For this review, take the finished solid that the model builds, in its own axes (mm). A direction names the side the tool comes from. Coordinates: 2 decimals unless noted, no trailing zeros. Loops run counter-clockwise (first coordinate to the right, second up) from the corner with the lowest first, then second, coordinate; pieces in that order, holes last. Notation, with made-up numbers: (48, -12.75) - (95, -12.75) arc R31 cw to (95, 26.25) - close; hole circle Ø11 at (9, 85). An arc over 180 degrees is marked (long way). One line per item, written item: value. Start each with the question number.
1. For faces 5 (the face through (37, 0, -5)), 6 (the face through (41, 0, -7.5)), 7 (the face through (37, 5, 0)), 8 (the face through (2.8, -8, 0)), 9 (the face through (7, 7, 2.5)), list the 3-axis set-ups (+Z, -Z, +X, -X, +Y, -Y) from which the entire face can be reached by the end or side of a thin tool; tool diameter is ignored.
2. Insertion check: pin 1 (2.5 mm diameter, centred on y = -8, z = 0.5, fed in from +X); pin 2 (4 mm diameter, centred on x = 17, y = 8.5, fed in from -Z); pin 3 (2.5 mm diameter, centred on x = 37.5, z = -0.5, fed in from -Y). Each pin has a flat end and moves straight along its axis. Give the tip position at first contact, or say it passes through.
3. Take a section at D-D, the plane x = 31.5. State the section outline as (y, z) points.
4. Take a section at A-A, the plane x = 0. State the section outline as (y, z) points.
5. Take a section at C-C, the plane y = 2. State the section outline as (x, z) points, and give its area (3 significant figures).
6. Take a section at B-B, the plane z = -1. State the section outline as (x, y) points.
7. The part is to be moulded in two halves that separate along X. For faces 1 (the face through (37, -5, 0)), 2 (the face through (-0.29, 7.494, 0.035)), 3 (the face through (-29.974, 1.249, 0.035)), 4 (the face through (-2.8, -9, 0)), say which applies: released by +X, released by -X, zero draft, split by the parting line, or undercut.
8. To check wall thickness, follow line 1 (Y direction, x = 0, z = -0.7); line 2 (X direction, y = 0, z = 1.4); line 3 (Y direction, x = 31.5, z = -1.5). State the ranges of each line that lie inside material, in increasing order. Write a range as from..to.
```python
from build123d import *

# Parameters (mm, degrees)
F1_DEPTH = 2.5
F2_R     = 4
F3_DEPTH = 5


with BuildPart() as f1:
    # F0 (on Top) → F1 (new body, symmetric)
    with BuildSketch(Plane.XY):
        with BuildLine():
            ThreePointArc((29.5803989155, -5), (29.8949156836, -2.5087878084), (30, 0))
            ThreePointArc((30, 0), (29.8949156836, 2.5087878084), (29.5803989155, 5))
            ThreePointArc((29.5803989155, 5), (-30, 0), (29.5803989155, -5))
        make_face()
        with BuildLine():
            ThreePointArc((-2.8, -6.9577295147), (-4.1982139059, 6.2149014473), (7.5, 0))
            ThreePointArc((7.5, 0), (6.2149014473, -4.1982139059), (2.8, -6.9577295147))
            Line((2.8, -6.9577295147), (2.8, -10))
            Line((2.8, -10), (0, -10))
            Line((0, -10), (-2.8, -10))
            Line((-2.8, -10), (-2.8, -6.9577295147))
        make_face(mode=Mode.SUBTRACT)
        with BuildLine():
            ThreePointArc((29.5803989155, 5), (29.8949156836, 2.5087878084), (30, 0))
            ThreePointArc((30, 0), (29.8949156836, -2.5087878084), (29.5803989155, -5))
            Line((29.5803989155, -5), (45, -5))
            Line((45, -5), (45, 0))
            Line((45, 0), (45, 5))
            Line((45, 5), (29.5803989155, 5))
        make_face()
    extrude(amount=F1_DEPTH, both=True)

    # F2 (on face) → F3 (join)
    with BuildSketch(Plane(origin=(0, 0, -2.5), x_dir=(1, 0, 0), z_dir=(0, 0, -1))):
        with Locations((41.0000477707, -0.0195490011)):
            Circle(F2_R)
    extrude(amount=F3_DEPTH)


solid = f1.part
```
Solutions:
1. face 5: -Z
1. face 6: -Z, +X, -X, +Y, -Y
1. face 7: +Z, -Z, +X, +Y
1. face 8: +Z, -Z
1. face 9: +Z, +X, -X, +Y, -Y
2. pin 1: x = 29.23
2. pin 2: z = -2.5
2. pin 3: y = -5
3. outline: (-5, -2.5) - (5, -2.5) - (5, 2.5) - (-5, 2.5) - close
4. outline: (-30, -2.5) - (-10, -2.5) - (-10, 2.5) - (-30, 2.5) - close; (7.5, -2.5) - (30, -2.5) - (30, 2.5) - (7.5, 2.5) - close
5. outline: (-29.93, -2.5) - (-7.23, -2.5) - (-7.23, 2.5) - (-29.93, 2.5) - close; (7.23, -2.5) - (37.52, -2.5) - (37.52, -7.5) - (44.48, -7.5) - (44.48, -2.5) - (45, -2.5) - (45, 2.5) - (7.23, 2.5) - close
5. area: 337 mm2
6. outline: (29.58, -5) - (45, -5) - (45, 5) - (29.58, 5) arc R30 ccw (long way) to start; hole (-2.8, -10) - (2.8, -10) - (2.8, -6.96) arc R7.5 ccw (long way) to (-2.8, -6.96) - close
7. face 1: zero draft
7. face 2: undercut
7. face 3: split by the parting line
7. face 4: undercut
8. line 1: -30..-10, 7.5..30
8. line 2: -30..-7.5, 7.5..45
8. line 3: -5..5
